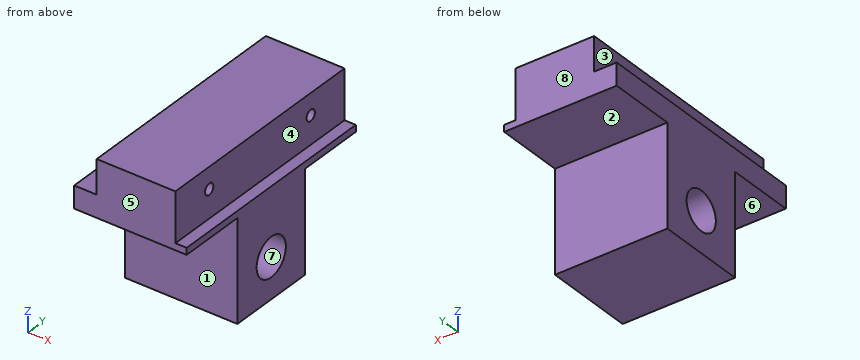
Solid Edge part; units mm, degrees
sketch "Sketch1" plane through (0, 0, 0) normal (0, -1, 0) x (1, 0, 0)
  line L0 (0, 0) -> (50, 0)
  line L1 (50, 0) -> (50, 3)
  line L2 (50, 3) -> (45, 3)
  line L3 (45, 3) -> (45, 25)
  line L4 (45, 25) -> (10, 25)
  line L5 (10, 25) -> (10, 24.85)
  line L6 (10, 24.85) -> (10, 9.85)
  line L7 (10, 9.85) -> (0, 9.85)
  line L8 (0, 9.85) -> (0, 0)
extrude "Protrusion1" add sketch "Sketch1" along normal mid plane 100
sketch "Sketch2" plane through (25, 0, 0) normal (0, 0, -1) x (1, 0, 0)
  line L0 (-25, -20) -> (25, -20)
  line L1 (25, -20) -> (25, 20)
  line L2 (25, 20) -> (-25, 20)
  line L3 (-25, 20) -> (-25, -20)
  dimension "D1" = 25
extrude "ExtrudedProtrusion_2" add sketch "Sketch2" along normal blind 45
hole "Hole_1" at (50, 0, -27) direction (-1, 0, 0) diameter 17.294 end through all
hole "Hole_8" at (45, -30, 15.5) direction (-1, 0, 0) diameter 4.917 depth 13 tip angle 118 thread major 6 thread length 10
hole "Hole1" at (45, 30, 15.5) direction (-1, 0, 0) diameter 4.917 depth 13 tip angle 118 thread major 6 thread length 10
properties part number "2" material "cast iron"
CAD build for the part. Positions are in the model's coordinates, mm. Face numbers are marked on the shaded views. A direction names the side the tool comes from. Give positions to 0.01 mm unless a question says otherwise; leave off trailing zeros. Write each loop counter-clockwise with the first axis right and the second up, starting at its lowest first coordinate (ties: lowest second). Pieces come first, ordered by that corner, then holes. Notation, with made-up numbers: M 49,75.25 L 95,75.25 A21 cw 95,106.25 Z; hole C 80,88 d9. An arc over 180 degrees is marked long. Put each result on its own line as item: value. Start each with the question number.
(1) Flat gauge pins, fed straight in: pin 1 Ø24 at (x, y) = (34.5, -33.5) entering from -Z; pin 2 Ø4.5 at (y, z) = (-14.5, 16.5) entering from -X; pin 3 Ø1 at (x, z) = (20.5, -8) entering from -Y. Where does each tip first touch, or does it go through?
(2) Which spindle directions (+Z, -Z, +X, -X, +Y, -Y) get a long thin tool onto all of the face, cutting with end or side? Do the marked faces 1, 2, 3, 4 and 5. Say none if no direction does.
(3) Band-saw the part on A-A, the plane x = 29. Write the cut outline in (y, z).
(4) Probe L1, parallel to Y at x = 36.25, z = 15.5; L2, parallel to Y at x = 17, z = -27; L3, parallel to X at y = 21.5, z = 22. List the from-to ranges inside material, lowest first.
(5) Mould opens along Y. For the marked faces 6, 7 and 8 say: +Y half, -Y half, draft (parallel to the pull), parting line (faces both ways), or undercut.
(6) Band-saw the part on B-B, the plane y = 0. Write the cut outline in (x, z).
(7) Band-saw the part on C-C, the plane x = 39. Write the cut outline in (y, z), and give its area (3 significant figures).
(8) Band-saw the part on D-D, the plane y = 40. Write the cut outline in (x, z).
Response values:
1. pin 1: stops at z = 0
1. pin 2: stops at x = 10
1. pin 3: stops at y = -20
2. face 1: -Z, +X, -X, -Y
2. face 2: -Z, +X, -X, +Y
2. face 3: +Z, -X, +Y, -Y
2. face 4: +Z, +X, +Y, -Y
2. face 5: +Z, -Z, +X, -X, -Y
3. outline: M -50,0 L -20,0 L -20,-45 L 20,-45 L 20,0 L 50,0 L 50,25 L -50,25 Z; hole C 0,-27 d17.29
4. L1: y = -50 to -32.46, -27.54 to 27.54, 32.46 to 50
4. L2: y = -20 to -8.65, 8.65 to 20
4. L3: x = 10 to 45
5. face 6: draft
5. face 7: undercut
5. face 8: +Y half
6. outline: M 0,-45 L 50,-45 L 50,-35.65 L 0,-35.65 Z; M 0,-18.35 L 50,-18.35 L 50,3 L 45,3 L 45,25 L 10,25 L 10,9.85 L 0,9.85 Z
7. outline: M -50,0 L -20,0 L -20,-45 L 20,-45 L 20,0 L 50,0 L 50,25 L -50,25 Z; hole C -30,15.5 d4.92; hole C 0,-27 d17.29; hole C 30,15.5 d4.92
7. area: 4,030 mm2
8. outline: M 0,0 L 50,0 L 50,3 L 45,3 L 45,25 L 10,25 L 10,9.85 L 0,9.85 Z
